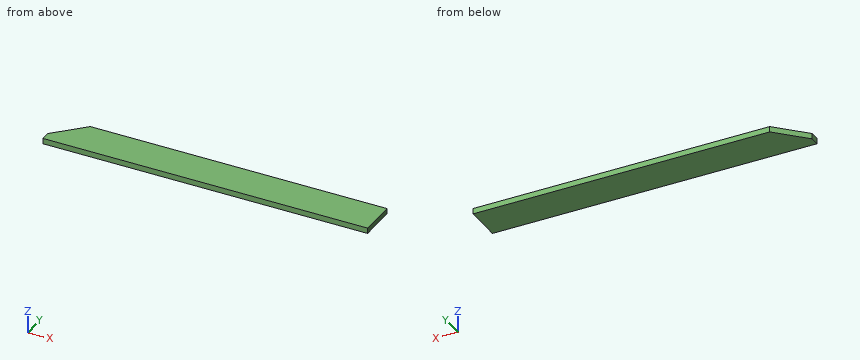
Autodesk Inventor part; units mm, degrees
ref_plane "YZ Plane" through (0, 0, 0) normal (1, 0, 0) x (0, 1, 0)
ref_plane "XZ Plane" through (0, 0, 0) normal (0, 1, 0) x (-1, 0, 0)
ref_plane "XY Plane" through (0, 0, 0) normal (0, 0, 1) x (1, 0, 0)
sketch "Sketch1" plane through (0, 0, 0) normal (0, 0, 1) x (1, 0, 0)
  line L0 (-175, 20) -> (0, 20)
  line L1 (0, 20) -> (0, 0)
  line L2 (0, 0) -> (-175, 0)
  line L3 (-175, 0) -> (-175, 20)
  dimension "d2" = 20
  dimension "d3" = 175
extrude "Plate1" add sketch "Sketch1" along normal mid plane 3
chamfer "Chamfer1" distance 15 angle 45 1 edges at (-175, 20, 0)
equation "\"d4\" = Thickness"
equation "\"BendReliefWidth\" = Thickness"
equation "\"BendReliefDepth\" = 0.5 * Thickness"
equation "\"CornerReliefSize\" = 4 * Thickness"
equation "\"MinimumRemnant\" = 2 * Thickness"
equation "\"TransitionRadius\" = BendRadius"
equation "\"JacobiRadiusSize\" = BendRadius"
equation "\"GapSize\" = Thickness"
properties part number "MSC 039 flange cover plate 500" material "Stainless Steel"
Design review of the part built by this model. Coordinates are the model's own, in mm. Coordinates: 2 decimals unless noted, no trailing zeros. Order: outer loops, then holes, each group sorted by start corner. A loop starts at its lowest first (then second) coordinate and runs counter-clockwise, first axis right, second up. Notation, with made-up numbers: M 35.25,7.25 L 71.25,7.25 A19 ccw 71.25,26.25 Z; hole C 6,7 d1. An arc over 180 degrees is marked long. Use a Markdown table: item, result.
(1) Wall thickness on probe 1 along X at (y, z) = (8.5, 0); probe 2 along X at (y, z) = (18, -0.4); probe 3 along Y at (x, z) = (-164.5, 0.9): over which ranges is each line inside the solid? List them lowest first.
Worked answers:
| item | result |
|---|---|
| probe 1 | x = -171.5 to 0 |
| probe 2 | x = -162 to 0 |
| probe 3 | y = 0 to 15.5 |
(2) Add section A-A (y = 17.5). Give the boundary of the cut face in (x, z), then the cut area to 4 significant figures.
Worked answers:
| item | result |
|---|---|
| outline | M -162.5,-1.5 L 0,-1.5 L 0,1.5 L -162.5,1.5 Z |
| area | 487.5 mm2 |
(3) Add section B-B (z = 0.5). Give the boundary of the cut face in (x, y), then the cut area to 3 significant figures.
Worked answers:
| item | result |
|---|---|
| outline | M -175,0 L 0,0 L 0,20 L -160,20 L -175,5 Z |
| area | 3,390 mm2 |
